Design review of the part built by this model. Coordinates are the model's own, in mm. A direction names the side the tool comes from. Coordinates: 2 decimals unless noted, no trailing zeros. Write each loop counter-clockwise with the first axis right and the second up, starting at its lowest first coordinate (ties: lowest second). Pieces come first, ordered by that corner, then holes. Notation, with made-up numbers: (0.5, 42) - (48.5, 42) arc R16 ccw to (48.5, 60) - close; hole circle Ø6 at (53.5, 41.25). An arc over 180 degrees is marked (long way). Answer as a JSON object with one key per item and string values.
```python
from build123d import *

# Parameters (mm, degrees)
IZIM1_R                                        = 68
Y_KSEKLIK_EKSTR_ZYON1_DEPTH                    = 5
IZIM2_W                                        = 42
IZIM2_H                                        = 32
Y_KSEKLIK_EKSTR_ZYON2_DEPTH                    = 16.3
IZIM3_W                                        = 32
IZIM3_H                                        = 32
KES_EKSTR_ZYON1_DEPTH                          = 11.3
M2_D_Z_BA_L_MAKINE_VIDAS_IN_HAV_A2_D           = 2
M2_D_Z_BA_L_MAKINE_VIDAS_IN_HAV_A2_CSINK_D     = 2.6
M2_D_Z_BA_L_MAKINE_VIDAS_IN_HAV_A2_CSINK_ANGLE = 90
IZIM9_W                                        = 6.3
IZIM9_H                                        = 20
KES_EKSTR_ZYON2_DEPTH                          = 151.005633228
RADYUS1_R                                      = 3
M2_D_Z_BA_L_MAKINE_VIDAS_IN_HAV_A3_D           = 2
M2_D_Z_BA_L_MAKINE_VIDAS_IN_HAV_A3_DEPTH       = 5
M2_D_Z_BA_L_MAKINE_VIDAS_IN_HAV_A3_CSINK_D     = 2.6
M2_D_Z_BA_L_MAKINE_VIDAS_IN_HAV_A3_CSINK_ANGLE = 90
AYNALAMA2_COPY_1_D                             = 2
AYNALAMA2_COPY_1_DEPTH                         = 5
AYNALAMA2_COPY_1_CSINK_D                       = 2.6
AYNALAMA2_COPY_1_CSINK_ANGLE                   = 90


with BuildPart() as part:
    # Çizim1 → Yükseklik-Ekstrüzyon1 (new body)
    with BuildSketch(Plane.XY):
        Circle(IZIM1_R)
    extrude(amount=Y_KSEKLIK_EKSTR_ZYON1_DEPTH)

    # Çizim2 → Yükseklik-Ekstrüzyon2 (add)
    with BuildSketch(Plane.XY.offset(5)):
        with Locations((-43, 0)):
            Rectangle(IZIM2_W, IZIM2_H)
        with Locations((43, 0)):
            Rectangle(IZIM2_W, IZIM2_H)
    extrude(amount=Y_KSEKLIK_EKSTR_ZYON2_DEPTH)

    # Çizim3 → Kes-Ekstrüzyon1 (cut)
    with BuildSketch(Plane.XY.offset(21.3)):
        with Locations((-43, 0)):
            Rectangle(IZIM3_W, IZIM3_H)
        with Locations((43, 0)):
            Rectangle(IZIM3_W, IZIM3_H)
    extrude(amount=-KES_EKSTR_ZYON1_DEPTH, mode=Mode.SUBTRACT)

    # M2 Düz Başlı Makine Vidası İçin Havşa2 (through all)
    with Locations(Plane(origin=(0, 8, 5), x_dir=(1, 0, 0), z_dir=(0, 0, 1))):
        with Locations((0, 0), (8, -8), (0, -16), (-8, -8)):
            CounterSinkHole(M2_D_Z_BA_L_MAKINE_VIDAS_IN_HAV_A2_D / 2, M2_D_Z_BA_L_MAKINE_VIDAS_IN_HAV_A2_CSINK_D / 2, counter_sink_angle=M2_D_Z_BA_L_MAKINE_VIDAS_IN_HAV_A2_CSINK_ANGLE)

    # Çizim9 → Kes-Ekstrüzyon2 (cut, through all)
    with BuildSketch(Plane(origin=(64, 0, 0), x_dir=(0, 0, -1), z_dir=(1, 0, 0))):
        with Locations((-18.15, 0)):
            Rectangle(IZIM9_W, IZIM9_H)
    extrude(amount=-KES_EKSTR_ZYON2_DEPTH, mode=Mode.SUBTRACT)

    # Radyus1
    radyus1_edges = [part.edges().sort_by_distance(p)[0] for p in [
        (-61.5, 10, 21.3),
        (-61.5, 16, 21.3),
        (61.5, -16, 21.3),
        (61.5, -10, 21.3),
        (24.5, -16, 21.3),
        (24.5, -10, 21.3),
        (61.5, 10, 21.3),
        (24.5, 10, 21.3),
        (24.5, 16, 21.3),
        (61.5, 16, 21.3),
        (-24.5, 10, 21.3),
        (-24.5, 16, 21.3),
        (-24.5, -16, 21.3),
        (-24.5, -10, 21.3),
        (-61.5, -16, 21.3),
        (-61.5, -10, 21.3),
    ]]
    fillet(radyus1_edges, radius=RADYUS1_R - 0.0001)  # a hair under: the kernel refuses the full size

    # M2 Düz Başlı Makine Vidası İçin Havşa3
    with Locations(Plane(origin=(64, 13.5, 18), x_dir=(0, 1, 0), z_dir=(1, 0, 0))):
        with Locations((0, 0), (-5.5, -5.5), (-21.5, -5.5), (-27, 0)):
            m2_d_z_ba_l_makine_vidas_in_hav_a3 = CounterSinkHole(M2_D_Z_BA_L_MAKINE_VIDAS_IN_HAV_A3_D / 2, M2_D_Z_BA_L_MAKINE_VIDAS_IN_HAV_A3_CSINK_D / 2, depth=M2_D_Z_BA_L_MAKINE_VIDAS_IN_HAV_A3_DEPTH, counter_sink_angle=M2_D_Z_BA_L_MAKINE_VIDAS_IN_HAV_A3_CSINK_ANGLE)

    # Aynalama1: M2 Düz Başlı Makine Vidası İçin Havşa3 across plane
    add(m2_d_z_ba_l_makine_vidas_in_hav_a3.mirror(Plane(origin=(43, 0, 0), x_dir=(0, 0, 1), z_dir=(1, 0, 0))), mode=Mode.SUBTRACT)

    # Aynalama2: M2 Düz Başlı Makine Vidası İçin Havşa3 across plane
    add(m2_d_z_ba_l_makine_vidas_in_hav_a3.mirror(Plane(origin=(0, 0, 0), x_dir=(0, 0, 1), z_dir=(1, 0, 0))), mode=Mode.SUBTRACT)

    # Aynalama2 copy 1
    with Locations(Plane(origin=(-22, 13.5, 18), x_dir=(0, 1, 0), z_dir=(1, 0, 0))):
        with Locations((0, 0), (-5.5, -5.5), (-21.5, -5.5), (-27, 0)):
            CounterSinkHole(AYNALAMA2_COPY_1_D / 2, AYNALAMA2_COPY_1_CSINK_D / 2, depth=AYNALAMA2_COPY_1_DEPTH, counter_sink_angle=AYNALAMA2_COPY_1_CSINK_ANGLE)


solid = part.part
```
(1) For pin 1 (4 mm diameter, centred on x = 25, z = 19, fed in from -Y); pin 2 (2.5 mm diameter, centred on y = 13.5, z = 18, fed in from +X); pin 3 (2.5 mm diameter, centred on x = -60.5, y = 3.5, fed in from +Z), all flat-tipped, find the tip position at first contact; note any pin that passes through.
Solved:
{"pin 1": "stops at y = -16", "pin 2": "stops at x = 63.95", "pin 3": "stops at z = 15"}
(2) To check wall thickness, follow line 1 (Y direction, x = 25.1, z = 18); line 2 (Y direction, x = -23.5, z = 12.5); line 3 (Y direction, x = 0, z = 3.45). State the ranges of each line that lie inside material, in increasing order. Write a range as from..to.
Solved:
{"line 1": "y = -16..-14.5, -12.5..-10, 10..12.5, 14.5..16", "line 2": "y = -16..-9, -7..7, 9..16", "line 3": "y = -68..-9, -7..7, 9..68"}
(3) Tool access review of faces 1 (the face through (-59, 0, 14)), 2 (the face through (43, 16, 9)), 3 (the face through (-43, -16, 9)), 4 (the face through (25, 0, 15)): name each direction out of +Z, -Z, +X, -X, +Y, -Y from which nothing blocks a thin tool from reaching the whole face with its end or side.
Solved:
{"face 1": "+Z, +Y, -Y", "face 2": "+Z, +X, -X, +Y", "face 3": "+Z, +X, -X, -Y", "face 4": "+Z, +X, -X"}
(4) Take a section at A-A, the plane z = 2.5. Write out the cut boundary in (x, y).
Solved:
{"outline": "circle Ø136 at (0, 0); hole circle Ø2 at (-8, 0); hole circle Ø2 at (0, -8); hole circle Ø2 at (0, 8); hole circle Ø2 at (8, 0)"}
(5) Take a section at D-D, the plane x = -36.5. Write out the cut boundary in (y, z).
Solved:
{"outline": "(-57.37, 0) - (57.37, 0) - (57.37, 5) - (16, 5) - (16, 10) - (-16, 10) - (-16, 5) - (-57.37, 5) - close"}
(6) Take a section at C-C, the plane y = -54. Write out the cut boundary in (x, z).
Solved:
{"outline": "(-41.33, 0) - (41.33, 0) - (41.33, 5) - (-41.33, 5) - close"}
(7) The part is to be moulded in two halves that separate along X. For faces 5 (the face through (-24, 0, 15)), 6 (the face through (36.556, 57.338, 2.465)), 7 (the face through (22, 0, 11)), say which applies: pulls with the +X half, pulls with the -X half, needs draft (parallel to the pull), parting line crosses it, or undercut.
Solved:
{"face 5": "needs draft", "face 6": "parting line crosses it", "face 7": "undercut"}
(8) Take a section at B-B, the plane x = 34. Write out the cut boundary in (y, z), and give its area (3 significant figures).
Solved:
{"outline": "(-58.89, 0) - (58.89, 0) - (58.89, 5) - (16, 5) - (16, 10) - (-16, 10) - (-16, 5) - (-58.89, 5) - close", "area": "749 mm^2"}
